from build123d import *

# Parameters (mm, degrees)
Y_KSEKLIK_EKSTR_ZYON1_DEPTH = 30
Y_KSEKLIK_EKSTR_ZYON2_DEPTH = 10
IZIM5_R                     = 190
Y_KSEKLIK_EKSTR_ZYON3_DEPTH = 20
Y_KSEKLIK_EKSTR_ZYON4_DEPTH = 13
DAIRESEL_KAPLAMA1_COUNT     = 20
IZIM7_R                     = 45
Y_KSEKLIK_EKSTR_ZYON5_DEPTH = 150
RADYUS1_R                   = 10


with BuildPart() as part:
    # Çizim1 → Yükseklik-Ekstrüzyon1 (new body)
    with BuildSketch(Plane.XY):
        with BuildLine():
            Line((-2560, 390), (-2560, 225))
            ThreePointArc((-2560, 225), (-2635, -150), (-2710, 225))
            Line((-2710, 225), (-2710, 390))
            Line((-2710, 390), (-2560, 390))
        make_face()
    extrude(amount=-Y_KSEKLIK_EKSTR_ZYON1_DEPTH)

    # Çizim4 → Yükseklik-Ekstrüzyon2 (add)
    with BuildSketch(Plane(origin=(0, 0, -30), x_dir=(-1, 0, 0), z_dir=(0, 0, -1))):
        with BuildLine():
            Line((2510, 390), (2510, 255.713075057))
            ThreePointArc((2510, 255.713075057), (2635, -200), (2760, 255.713075057))
            Line((2760, 255.713075057), (2760, 390))
            Line((2760, 390), (2510, 390))
        make_face()
    extrude(amount=Y_KSEKLIK_EKSTR_ZYON2_DEPTH)

    # Çizim5 → Yükseklik-Ekstrüzyon3 (add)
    with BuildSketch(Plane(origin=(0, 0, -40), x_dir=(-1, 0, 0), z_dir=(0, 0, -1))):
        with Locations((2635, 45)):
            Circle(IZIM5_R)
    extrude(amount=Y_KSEKLIK_EKSTR_ZYON3_DEPTH)

    # Çizim6 → Yükseklik-Ekstrüzyon4 (add)
    with BuildSketch(Plane(origin=(0, 0, -40), x_dir=(-1, 0, 0), z_dir=(0, 0, -1))):
        Polygon((2639.970562748, 250.5), (2647, 257.529437252), (2647, 267.470562748), (2639.970562748, 274.5), (2630.029437252, 274.5), (2623, 267.470562748), (2623, 257.529437252), (2630.029437252, 250.5), align=None)
    y_kseklik_ekstr_zyon4 = extrude(amount=Y_KSEKLIK_EKSTR_ZYON4_DEPTH)

    # Dairesel Kaplama1: Yükseklik-Ekstrüzyon4 ×20 about axis
    dairesel_kaplama1_axis = Axis((-2635, 45, 0), (0, 0, 1))
    for i in range(1, DAIRESEL_KAPLAMA1_COUNT):
        add(y_kseklik_ekstr_zyon4.rotate(dairesel_kaplama1_axis, i * 360 / DAIRESEL_KAPLAMA1_COUNT))

    # Çizim7 → Yükseklik-Ekstrüzyon5 (add)
    with BuildSketch(Plane(origin=(0, 0, -60), x_dir=(-1, 0, 0), z_dir=(0, 0, -1))):
        with Locations((2635, 45)):
            Circle(IZIM7_R)
    extrude(amount=Y_KSEKLIK_EKSTR_ZYON5_DEPTH)

    # Radyus1
    radyus1_edges = [part.edges().sort_by_distance(p)[0] for p in [
        (-2590, 45, -60),
        (-2590, 45, -210),
    ]]
    fillet(radyus1_edges, radius=RADYUS1_R)


solid = part.part
Could you check a few things on this model? Use its own coordinates, in mm. A direction names the side the tool comes from. Give positions to 0.01 mm unless a question says otherwise; leave off trailing zeros. Write each loop counter-clockwise with the first axis right and the second up, starting at its lowest first coordinate (ties: lowest second). Pieces come first, ordered by that corner, then holes. Notation, with made-up numbers: (60.5, 88) -> (98.5, 88) arc R14 cw to (98.5, 97) -> close; hole circle Ø3 at (29.5, -21.5). An arc over 180 degrees is marked (long way). Answer as CSV lines item,"result". Start each with the question number.
(1) Which directions (+Z, -Z, +X, -X, +Y, -Y) give clear straight access to the entire face, cutting with the end or side of a thin tool? Please do faces 1 (the face through (-2811, 173, -53)), 2 (the face through (-2452, 118, -30)), 3 (the face through (-2635, 263, -53)), 4 (the face through (-2417, 45, -53)), 5 (the face through (-2842, 112, -53)).
(2) I'm going to push flat-ended pins straight in: pin 1 Ø10 at (x, z) = (-2650, -77) entering from -Y; pin 2 Ø24 at (y, z) = (322, -18.5) entering from -X; pin 3 Ø8 at (x, y) = (-2429, -17) entering from -Z. Where does each tip first touch, or does it pass through?
(3) Please list where these lines run through material, in increasing order: line 1 (Z direction, x = -2721, y = 26); line 2 (Z direction, x = -2574.5, y = 339); line 3 (X direction, y = 14, z = -117).
(4) If we mould it in two halves opening along X, with no side actions, what happens to faces 6 (the face through (-2627.503, -149.856, -14.79)), 7 (the face through (-2811, -83, -53)), 8 (the face through (-2634, 249, -40))? For each: +X half, -X half, draft (parallel to the pull), parting line (faces both ways), or undercut.
(5) If we section it at A-A, the plane z = -127: Write out the boundary of the cut face in (x, y).
Answer list:
1,face 1,"-Z, -X, +Y"
1,face 2,"+Z"
1,face 3,"-Z, +X, -X, +Y"
1,face 4,"-Z, +X, +Y, -Y"
1,face 5,"-Z, -X, +Y, -Y"
2,pin 1,"y = 1.13"
2,pin 2,"x = -2760"
2,pin 3,"z = -53"
3,line 1,"-60 to 0"
3,line 2,"-40 to 0"
3,line 3,"-2667.62 to -2602.38"
4,face 6,"parting line"
4,face 7,"draft"
4,face 8,"undercut"
5,outline,"circle Ø90 at (-2635, 45)"
